```python
from build123d import *

# Parameters (mm, degrees)
F0_R     = 3.175
F0_W     = 9.525
F0_H     = 12.7
F1_DEPTH = 1.7145
F2_R     = 4.7625
F3_DEPTH = 63.5
F4_R     = 3.175
F5_DEPTH = 63.501
F6_W     = 12.38743
F6_H     = 12.7
F6_W_2   = 12.611339
F7_DEPTH = 25.4


with BuildPart() as f1:
    # F0 (on Front) → F1 (new body)
    with BuildSketch(Plane.XZ):
        Polygon((0, 12.7), (0, 0), (25.4, 0), (25.4, 63.5), (0, 63.5), (0, 50.8), (0, 38.1), (0, 25.4), align=None)
        with Locations((15.875, 12.7)):
            Circle(F0_R, mode=Mode.SUBTRACT)
        with Locations((15.875, 31.75)):
            Circle(F0_R, mode=Mode.SUBTRACT)
        with Locations((15.875, 50.8)):
            Circle(F0_R, mode=Mode.SUBTRACT)
        with Locations((-4.7625, 6.35)):
            Rectangle(F0_W, F0_H)
        with Locations((-4.7625, 31.75)):
            Rectangle(F0_W, F0_H)
        with Locations((-4.7625, 57.15)):
            Rectangle(F0_W, F0_H)
    extrude(amount=F1_DEPTH)

    # F2 (on face) → F3 (join)
    with BuildSketch(Plane.XY.offset(63.5)):
        with Locations((-6.35, 3.048)):
            Circle(F2_R)
    extrude(amount=-F3_DEPTH)

    # F4 (on face) → F5 (cut, through all)
    with BuildSketch(Plane.XY.offset(63.5)):
        with BuildLine():
            ThreePointArc((-6.35, -1.7145), (-8.049365, -1.400996), (-9.525, -0.501758))
            Line((-9.525, -0.501758), (-9.525, -1.7145))
            Line((-9.525, -1.7145), (-6.35, -1.7145))
        make_face()
        with Locations((-6.35, 3.048)):
            Circle(F4_R)
    extrude(amount=-F5_DEPTH, mode=Mode.SUBTRACT)

    # F6 (on face) → F7 (cut)
    with BuildSketch(Plane.XZ.offset(1.7145)):
        with Locations((-6.193715, 44.45)):
            Rectangle(F6_W, F6_H)
        with Locations((-6.305669, 19.05)):
            Rectangle(F6_W_2, F6_H)
    extrude(amount=-F7_DEPTH, mode=Mode.SUBTRACT)


solid = f1.part
```
Input: part model. Units: mm. Frame: model coordinates. A direction names the side the tool comes from. Coordinates: 2 decimals unless noted, no trailing zeros. Loops run counter-clockwise (first coordinate to the right, second up) from the corner with the lowest first, then second, coordinate; pieces in that order, holes last. Notation, with made-up numbers: M 6.5,79.25 L 26.5,79.25 A27 ccw 26.5,112.25 Z; hole C -19.5,-9 d9. An arc over 180 degrees is marked long. Use a Markdown table: item, result. Add a question column.
1) Section C-C, the plane x = -4.5. Return the cut outline in (y, z).
2) Set-up query: faces 1 (the flat face through (0, -1, 45)), 2 (the flat face through (9, -1.714, 32)). Return all of +Z, -Z, +X, -X, +Y, -Y with unobstructed straight access to the full face (end or side cutting, diameter ignored); none if empty.
3) Section B-B, the plane y = 5.5. Return the cut outline in (x, z), plus the area to 3 significant figures.
4) Draft query along Z for faces 3 (the flat face through (3, -1, 0)), 4 (the flat face through (-5.6, -0.2, 12.7)), 5 (the cylindrical face through (-4.885, 0.231, 57.239)). Return one class per face: +Z half, -Z half, draft (parallel to the pull), parting line (faces both ways), or undercut.
5) Line query: L1, parallel to Z at x = -6, y = 6.75; L2, parallel to Z at x = 13, y = -0.5; L3, parallel to X at y = 3, z = 54. Output: solid intervals per line, ascending. Write a range as from..to.
6) Section A-A, the plane z = 31.75. Give the number of separate pieces and of enclosed holes in the cut face, plus the area to 3 significant figures.
7) Pin query (flat end, axial travel): P1, Ø3, axis at x = -7.5, y = 3, coming from the +Z side; P2, Ø5, axis at y = 2, z = 17.5, coming from the -X side; P3, Ø4, axis at y = 6.5, z = 38, coming from the +X side; P4, Ø8.5, axis at x = 17, z = 39.5, coming from the +Y side. Return the tip coordinate at first contact, or that it passes through.
Answer below:
| question | item | result |
|---|---|---|
| 1 | outline | M -1.71,0 L 0.47,0 L 0.47,12.7 L -1.71,12.7 Z; M -1.71,25.4 L 0.47,25.4 L 0.47,38.1 L -1.71,38.1 Z; M -1.71,50.8 L 0.47,50.8 L 0.47,63.5 L -1.71,63.5 Z; M 5.63,0 L 7.44,0 L 7.44,12.7 L 5.63,12.7 Z; M 5.63,25.4 L 7.44,25.4 L 7.44,38.1 L 5.63,38.1 Z; M 5.63,50.8 L 7.44,50.8 L 7.44,63.5 L 5.63,63.5 Z |
| 2 | face 1 | -X, +Y, -Y |
| 2 | face 2 | +Z, -Z, +X, -X, -Y |
| 3 | outline | M -10.43,0 L -8.37,0 L -8.37,12.7 L -10.43,12.7 Z; M -10.43,25.4 L -8.37,25.4 L -8.37,38.1 L -10.43,38.1 Z; M -10.43,50.8 L -8.37,50.8 L -8.37,63.5 L -10.43,63.5 Z; M -4.33,0 L -2.27,0 L -2.27,12.7 L -4.33,12.7 Z; M -4.33,25.4 L -2.27,25.4 L -2.27,38.1 L -4.33,38.1 Z; M -4.33,50.8 L -2.27,50.8 L -2.27,63.5 L -4.33,63.5 Z |
| 3 | area | 157 mm2 |
| 4 | face 3 | -Z half |
| 4 | face 4 | undercut |
| 4 | face 5 | draft |
| 5 | L1 | 0..12.7, 25.4..38.1, 50.8..63.5 |
| 5 | L2 | 0..11.35, 14.05..30.4, 33.1..49.45, 52.15..63.5 |
| 5 | L3 | -11.11..-9.52, -3.18..-1.59 |
| 6 | separate pieces | 2 |
| 6 | enclosed holes | 1 |
| 6 | area | 78.8 mm2 |
| 7 | P1 | through |
| 7 | P2 | x = 0 |
| 7 | P3 | x = -1.81 |
| 7 | P4 | y = 0 |
